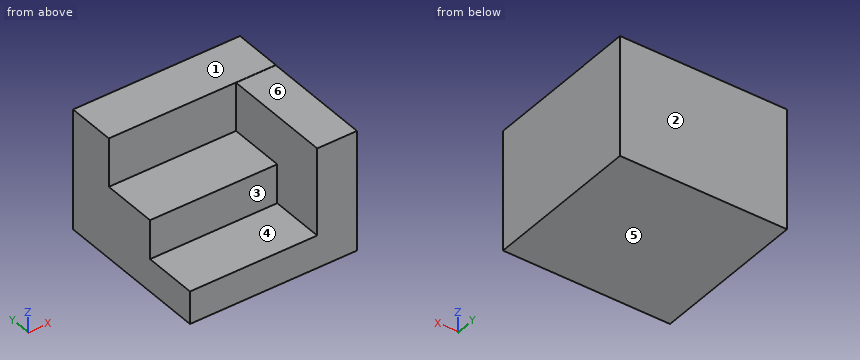
Solid Edge part; units mm, degrees
sketch "Sketch1" plane through (0, 0, 0) normal (-1, 0, 0) x (0, -1, 0)
  line L0 (9.9031, 22.7779) -> (21.3114, 22.7779)
  line L1 (21.3114, 22.7779) -> (21.3114, 14.8186)
  line L2 (21.3114, 14.8186) -> (32.366, 14.8186)
  line L3 (32.366, 14.8186) -> (32.366, 0)
  line L4 (32.366, 0) -> (0, 0)
  line L5 (0, 0) -> (0, 32.6828)
  line L6 (0, 32.6828) -> (9.9031, 32.6828)
  line L7 (9.9031, 32.6828) -> (9.9031, 22.7779)
extrude "Protrusion1" add sketch "Sketch1" against normal blind 34.0516
sketch "Sketch2" plane through (17.0258, -26.8387, 14.8186) normal (0, 0, 1) x (0, -1, 0)
  line L0 (5.5273, 8.9153) -> (5.5273, 17.0258)
  line L1 (5.5273, 17.0258) -> (-26.8387, 17.0258)
  line L2 (-26.8387, 17.0258) -> (-26.8387, 8.9153)
  line L3 (-26.8387, 8.9153) -> (5.5273, 8.9153)
extrude "ExtrudedProtrusion_2" add sketch "Sketch2" along normal blind 17.8195
sketch "Sketch3" plane through (17.0258, -32.366, 16.319) normal (0, -1, 0) x (1, 0, 0)
  line L0 (17.0258, -8.1568) -> (-17.0258, -8.1568)
  line L1 (-17.0258, -8.1568) -> (-17.0258, -16.319)
  line L2 (-17.0258, -16.319) -> (17.0258, -16.319)
  line L3 (17.0258, -16.319) -> (17.0258, -8.1568)
extrude "ExtrudedCutout_1" cut sketch "Sketch3" against normal blind 75.3715
The model under review builds one solid part; all positions refer to its coordinate system, in mm. Face numbers are marked on the shaded views. A direction names the side the tool comes from. Give positions to 0.01 mm unless a question says otherwise; leave off trailing zeros. Write each loop counter-clockwise with the first axis right and the second up, starting at its lowest first coordinate (ties: lowest second). Pieces come first, ordered by that corner, then holes. Notation, with made-up numbers: (30.5, 78.5) -> (61.5, 78.5) arc R14 cw to (61.5, 103.5) -> close; hole circle Ø5 at (47, 36.5). An arc over 180 degrees is marked (long way). Put each result on its own line as item: value.
(1) We need section C-C, the plane y = -28. Give the boundary of the cut face in (x, z).
Results are:
outline: (0, 8.16) -> (34.05, 8.16) -> (34.05, 32.64) -> (25.94, 32.64) -> (25.94, 14.82) -> (0, 14.82) -> close
(2) The part is to be moulded in two halves that separate along Y. For the marked faces 1, 2 and 3, say which applies: pulls with the +Y half, pulls with the -Y half, needs draft (parallel to the pull), parting line crosses it, or undercut.
Results are:
face 1: needs draft
face 2: pulls with the +Y half
face 3: pulls with the -Y half
(3) For pin 1 Ø5.5 at (x, y) = (17, -27.5) entering from +Z; pin 2 Ø2.5 at (x, y) = (28, -23.5) entering from +Z; pin 3 Ø3 at (x, z) = (16, 27) entering from -Y, all flat-tipped, find the tip position at first contact; note any pin that passes through.
Results are:
pin 1: z = 14.82
pin 2: z = 32.64
pin 3: y = -9.9
(4) To check wall thickness, follow probe 1 along Y at (x, z) = (12, 29.25); probe 2 along Y at (x, z) = (12.5, 19); probe 3 along Z at (x, y) = (11, -14.5). State the ranges of each line that lie inside material, in increasing order. Write a range as from..to.
Results are:
probe 1: -9.9..0
probe 2: -21.31..0
probe 3: 8.16..22.78
(5) Tool access review of the marked faces 4, 5 and 6: name each direction out of +Z, -Z, +X, -X, +Y, -Y from which nothing blocks a thin tool from reaching the whole face with its end or side.
Results are:
face 4: +Z, -X, -Y
face 5: -Z, +X, -X, +Y, -Y
face 6: +Z, +X, -X, -Y
(6) We need section A-A, the plane x = 4. Give the boundary of the cut face in (y, z).
Results are:
outline: (-32.37, 8.16) -> (0, 8.16) -> (0, 32.68) -> (-9.9, 32.68) -> (-9.9, 22.78) -> (-21.31, 22.78) -> (-21.31, 14.82) -> (-32.37, 14.82) -> close
(7) We need section B-B, the plane z = 16.25. Give the boundary of the cut face in (x, y).
Results are:
outline: (0, -21.31) -> (25.94, -21.31) -> (25.94, -32.37) -> (34.05, -32.37) -> (34.05, 0) -> (0, 0) -> close
